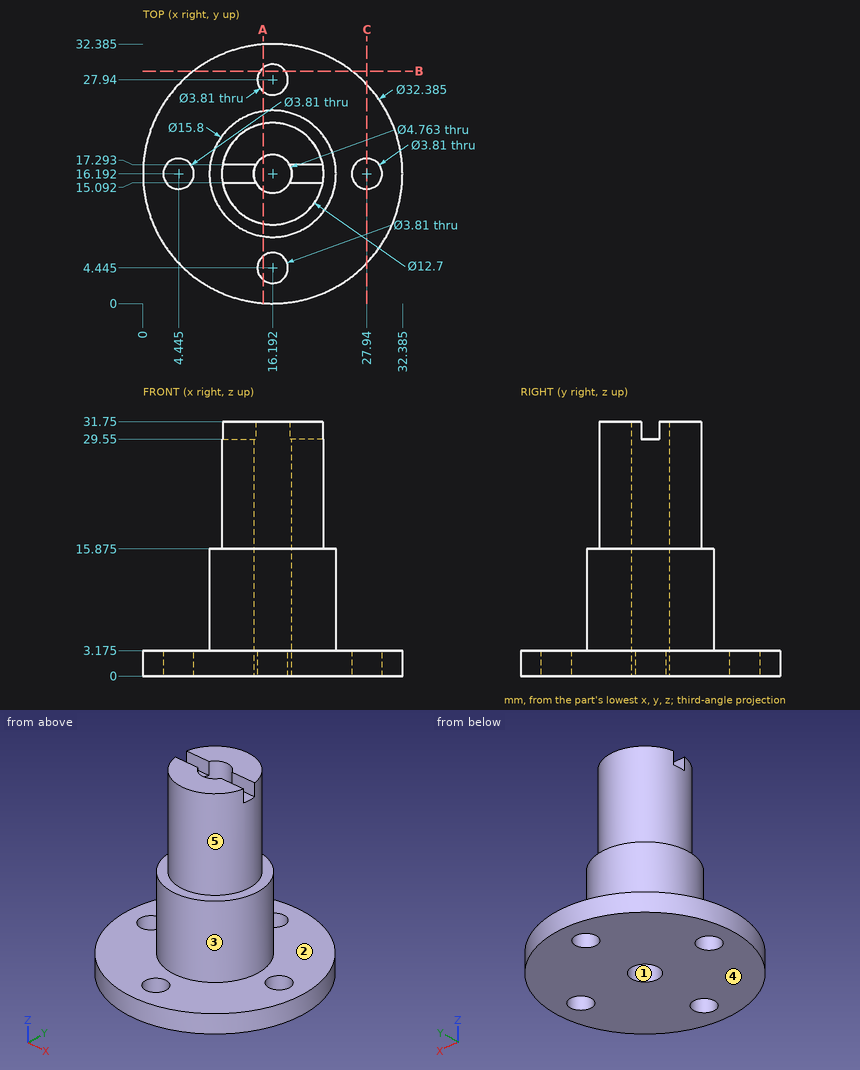
Can you work these out from the drawing? Everything is in mm from the part's minimum corner. A direction names the side the tool comes from. Round coordinates to 2 decimals unless told otherwise and drop trailing zeros. Loops run counter-clockwise (first coordinate to the right, second up) from the corner with the lowest first, then second, coordinate; pieces in that order, holes last. Notation, with made-up numbers: (73.5, 88.5) - (92.5, 88.5) arc R20 ccw to (92.5, 111.5) - close; hole circle Ø5 at (55, 85). An arc over 180 degrees is marked (long way). Answer in a Markdown table with one row per item. Add a question column.
(1) If we section it at A-A (x = 15): State how many separate pieces and enclosed holes the cut face has, plus the area to 3 significant figures.
(2) If we section it at C-C (x = 27.94): Please give me the cut outline in (y, z) (1 decimal).
(3) For the marked faces 4 and 5, which set-ups out of +Z, -Z, +X, -X, +Y, -Y let a thin tool reach every point of the face, with its end or its side?
(4) I'm going to push flat-ended pins straight in: pin 1 (10 mm diameter, centred on x = 10, y = 28.5, fed in from +Z) (1 decimal); pin 2 (1.8 mm diameter, centred on x = 21, z = 31, fed in from -Y); pin 3 (5 mm diameter, centred on y = 18, z = 16, fed in from +X). Where does each tip first touch, or does it pass through?
(5) I need wall thicknesses on line 1 along Y through (x, z) = (16, 6.5) (1 decimal); line 2 along Z through (x, y) = (20.5, 5.5) (1 decimal); line 3 along X through (y, z) = (16, 23.5) (1 decimal). Which ranges of each line are inside material? Lowest first, please.
(6) If we section it at B-B (y = 29): Please give me the cut outline in (x, z) (1 decimal).
(7) If we mould it in two halves opening along Y, with no side actions, what happens to the marked faces 1, 2 and 3? For each: pulls with the +Y half, pulls with the -Y half, needs draft (parallel to the pull), parting line crosses it, or undercut.
Model answer:
| question | item | result |
|---|---|---|
| 1 | separate pieces | 4 |
| 1 | enclosed holes | 0 |
| 1 | area | 349 mm² |
| 2 | outline | (5, 0) - (14.3, 0) - (14.3, 3.2) - (5, 3.2) - close; (18.1, 0) - (27.3, 0) - (27.3, 3.2) - (18.1, 3.2) - close |
| 3 | face 4 | -Z, +X, -X, +Y, -Y |
| 3 | face 5 | +Z |
| 4 | pin 1 | stops at z = 3.2 |
| 4 | pin 2 | stops at y = 11.19 |
| 4 | pin 3 | stops at x = 24.09 |
| 5 | line 1 | y = 8.3 to 13.8, 18.6 to 24.1 |
| 5 | line 2 | z = 0 to 3.2 |
| 5 | line 3 | x = 9.8 to 13.8, 18.6 to 22.5 |
| 6 | outline | (6.3, 0) - (14.6, 0) - (14.6, 3.2) - (6.3, 3.2) - close; (17.8, 0) - (26.1, 0) - (26.1, 3.2) - (17.8, 3.2) - close |
| 7 | face 1 | undercut |
| 7 | face 2 | needs draft |
| 7 | face 3 | parting line crosses it |
